Autodesk Inventor part; units mm, degrees
ref_plane "YZ Plane" through (0, 0, 0) normal (1, 0, 0) x (0, 1, 0)
ref_plane "XZ Plane" through (0, 0, 0) normal (0, 1, 0) x (-1, 0, 0)
ref_plane "XY Plane" through (0, 0, 0) normal (0, 0, 1) x (1, 0, 0)
sketch "Sketch1" plane through (0, 0, 0) normal (0, 1, 0) x (-1, 0, 0)
  line L0 (0, 0) -> (60, 0) construction
  line L1 (60, 0) -> (60, -20) construction
  line L2 (60, -20) -> (0, -20) construction
  line L3 (0, -20) -> (0, 0) construction
  line L4 (60.5, 0.5) -> (-0.5, 0.5)
  line L5 (-0.5, 0.5) -> (-0.5, -20.5)
  line L6 (-0.5, -20.5) -> (60.5, -20.5)
  line L7 (60.5, -20.5) -> (60.5, 0.5)
  circle A0 centre (53, -10) radius 1.8
  circle A1 centre (7, -10) radius 1.8
  line L8 (53, -10) -> (7, -10) construction
  point P0 (30, -10)
  point P1 (30, -20)
  point P2 (7, -10)
  point P3 (0, -10)
  dimension "d0" = 20
  dimension "d1" = 60
  dimension "d2" = 0.5
  dimension "d3" = 0.5
  dimension "d4" = 0.5
  dimension "d5" = 0.5
  dimension "d6" = 3.6
  dimension "d7" = 46
sketch "Sketch2" plane through (0, 0, 0) normal (0, 1, 0) x (-1, 0, 0)
  line L0 (-5.4, 7.5) -> (65.4, 7.5)
  line L1 (65.4, 7.5) -> (65.4, -27.5)
  line L2 (65.4, -27.5) -> (-5.4, -27.5)
  line L3 (-5.4, -27.5) -> (-5.4, 7.5)
  line L4 (60.5, -20.5) -> (60.5, 0.5) construction
  line L5 (-0.5, 0.5) -> (-0.5, -20.5) construction
  line L6 (-0.5, -20.5) -> (60.5, -20.5) construction
  point P0 (0, 0)
  point P1 (60.5, -10)
  point P2 (65.4, -10)
  point P3 (30, -20.5)
  point P4 (30, -27.5)
  dimension "d9" = 70.8
  dimension "d10" = 35
extrude "Extrusion1" add sketch "Sketch2" along normal blind 10 and the other way blind 35.4
extrude "Extrusion2" cut sketch "Sketch1" along normal blind 10 and the other way blind 2
extrude "Extrusion3" cut sketch "Sketch1" along normal blind 10 and the other way blind 30.4 contours A0 | A1
sketch "Sketch3" plane through (5.4, 10, -27.5) normal (0, 0, -1) x (-1, 0, 0)
  line L0 (70.8, -45.4) -> (0, -45.4)
  line L1 (0, -45.4) -> (0, -75.4)
  line L2 (0, -75.4) -> (10, -75.4)
  line L3 (10, -75.4) -> (10, -48.575)
  line L4 (13.175, -45.4) -> (57.625, -45.4)
  line L5 (60.8, -48.575) -> (60.8, -75.4)
  line L6 (60.8, -75.4) -> (70.8, -75.4)
  line L7 (70.8, -75.4) -> (70.8, -45.4)
  arc A0 (13.175, -45.4) -> (10, -48.575) centre (13.175, -48.575) ccw
  arc A1 (60.8, -48.575) -> (57.625, -45.4) centre (57.625, -48.575) ccw
  point P0 (5.4, -10)
  point P1 (10, -45.4)
  point P2 (60.8, -45.4)
  point P3 (35.4, -45.4)
  point P4 (13.175, -45.4)
  point P5 (57.625, -45.4)
  dimension "d23" = 50.8
  dimension "d24" = 3.175
  dimension "d25" = 10
  dimension "d26" = 30
extrude "Extrusion4" add sketch "Sketch3" against normal up to surface (35 mm away)
sketch "Sketch4" plane through (0, -2, 0) normal (0, 1, 0) x (1, 0, 0)
  circle A0 centre (-42.5, 10) radius 3
  circle A1 centre (-17.5, 10) radius 3
  line L0 (-60.5, 20.5) -> (0.5, 20.5) construction
  line L1 (-60.5, -0.5) -> (-60.5, 20.5) construction
  line L2 (-42.5, 10) -> (-17.5, 10) construction
  point P0 (0, 0)
  point P1 (-30, 20.5)
  point P2 (-30, 10)
  point P3 (-60.5, 10)
  dimension "d29" = 6
  dimension "d30" = 25
extrude "Extrusion5" cut sketch "Sketch4" against normal up to surface (33.4 mm away)
sketch "Sketch5" plane through (0, -2, 0) normal (0, 1, 0) x (1, 0, 0)
  circle A0 centre (-42.5, 10) radius 3 construction
  circle A1 centre (-17.5, 10) radius 3 construction
  circle A2 centre (-17.5, 10) radius 6
  circle A3 centre (-42.5, 10) radius 6
  point P0 (0, 0)
  dimension "d34" = 12
extrude "Extrusion6" cut sketch "Sketch5" against normal blind 10
fillet "Fillet1" radius 2 2 edges at (-65.4, 10, -10) (5.4, 10, -10)
fillet "Fillet2" radius 2 2 edges at (-65.4, -65.4, -10) (5.4, -65.4, -10)
properties part number "BK12_Spacer"
Check sheet for the modelled part. Datum: model origin and axes. Units: mm. A direction names the side the tool comes from. Coordinates: 2 decimals unless noted, no trailing zeros. Loops run counter-clockwise (first coordinate to the right, second up) from the corner with the lowest first, then second, coordinate; pieces in that order, holes last.
1) Release check for a two-part mould opening along Z. For faces 1 (the face through (-54.49, -36.35, -10.24)), 2 (the face through (-30, -2, -10)), 3 (the face through (-30, -20, -27.5)) record: released by +Z, released by -Z, zero draft, split by the parting line, or undercut.
2) Sectioned sample at C-C (z = -23.5). Record the boundary of the cut face in (x, y) (3 decimals).
3) Material ranges on probe 1 along X at (y, z) = (-52, -18.5); probe 2 along X at (y, z) = (7, -11); probe 3 along Z at (x, y) = (-17.5, -25.5), recorded low to high.
4) Access from +Z, -Z, +X, -X, +Y, -Y to the whole of each face (thin tool, end or side, straight path). Record for faces 4 (the face through (-4.6, -52, -10)), 5 (the face through (-6.61, -16.001, -11.757)), 6 (the face through (-59, -65.4, -10)).
5) Gauge pin test, flat ends, axial feed: pin 1 (6.5 mm diameter, centred on x = -35, z = -9, fed in from +Y); pin 2 (8 mm diameter, centred on x = -42.5, z = -10, fed in from -Y); pin 3 (3 mm diameter, centred on x = -7, z = -10, fed in from -Y). Record the tip position at first contact, or that the pin passes through.
6) Sectioned sample at D-D (x = -58.5). Record the boundary of the cut face in (y, z).
7) Sectioned sample at B-B (y = -59). Record the boundary of the cut face in (x, z), and give its area (3 significant figures).
8) Sectioned sample at A-A (x = -42.5). Record the boundary of the cut face in (y, z), and give its area (3 significant figures).
Check sheet entries:
1. face 1: zero draft
1. face 2: undercut
1. face 3: released by -Z
2. outline: (-65.4, -63.4) arc R2 ccw to (-63.4, -65.4) - (-55.4, -65.4) - (-55.4, -38.575) arc R3.175 cw to (-52.225, -35.4) - (-7.775, -35.4) arc R3.175 cw to (-4.6, -38.575) - (-4.6, -65.4) - (3.4, -65.4) arc R2 ccw to (5.4, -63.4) - (5.4, 8) arc R2 ccw to (3.4, 10) - (-63.4, 10) arc R2 ccw to (-65.4, 8) - close
3. probe 1: x = -65.4 to -55.4, -4.6 to 5.4
3. probe 2: x = -65.4 to -60.5, 0.5 to 5.4
3. probe 3: z = -27.5 to -13, -7 to 7.5
4. face 4: +Z, -Z, -Y
4. face 5: +Y
4. face 6: +Z, -Z, +X, -X, -Y
5. pin 1: stops at y = -2
5. pin 2: stops at y = -35.4
5. pin 3: stops at y = -36.36
6. outline: (-65.4, -27.5) - (10, -27.5) - (10, -20.5) - (-2, -20.5) - (-2, 0.5) - (10, 0.5) - (10, 7.5) - (-65.4, 7.5) - close
7. outline: (-65.4, -27.5) - (-55.4, -27.5) - (-55.4, 7.5) - (-65.4, 7.5) - close; (-4.6, -27.5) - (5.4, -27.5) - (5.4, 7.5) - (-4.6, 7.5) - close
7. area: 700 mm2
8. outline: (-35.4, -27.5) - (10, -27.5) - (10, -20.5) - (-2, -20.5) - (-2, -16) - (-12, -16) - (-12, -13) - (-35.4, -13) - close; (-35.4, -7) - (-12, -7) - (-12, -4) - (-2, -4) - (-2, 0.5) - (10, 0.5) - (10, 7.5) - (-35.4, 7.5) - close
8. area: 1,080 mm2
